Verification items for the finished model (mm, model axes). Face numbers are marked on the shaded views. A direction names the side the tool comes from. Give positions to 0.01 mm unless a question says otherwise; leave off trailing zeros. Write each loop counter-clockwise with the first axis right and the second up, starting at its lowest first coordinate (ties: lowest second). Pieces come first, ordered by that corner, then holes. Notation, with made-up numbers: (19, 77.5) - (38, 77.5) arc R28 cw to (38, 104.5) - close; hole circle Ø9 at (12, 24). An arc over 180 degrees is marked (long way). Answer as a JSON object with one key per item and string values. Group by question number.
Item 1: Draft check along Z on the marked faces 5, 6 and 7. Enter one of: +Z half, -Z half, draft (parallel to the pull), parting line (faces both ways), or undercut.
Item 2: Sectioned sample at C-C, the plane z = 15.5. Record the boundary of the cut face in (x, y), and give its area (3 significant figures).
Item 3: Sectioned sample at A-A, the plane x = 33. Record the boundary of the cut face in (y, z), and give its area (3 significant figures).
Item 4: Go/stop test with flat-tipped pins: pin 1 (5 mm diameter, centred on x = -39, y = 11, fed in from -Z); pin 2 (20 mm diameter, centred on y = 14.5, z = 8.5, fed in from +X); pin 3 (5 mm diameter, centred on y = 32, z = 1.5, fed in from -X). Record where each tip stops, or that it passes through.
Item 5: Sectioned sample at B-B, the plane y = 7.5. Record the boundary of the cut face in (x, z).
Item 6: Sectioned sample at D-D, the plane x = 19. Record the boundary of the cut face in (y, z).
Item 7: Tool access check on the marked faces 1, 2, 3 and 4. Record the directions out of +Z, -Z, +X, -X, +Y, -Y that give a thin tool (end or side, any length) a straight path to the whole face; none if there is none.
Item 8: Scan lines: line 1 along Z through (x, y) = (29, 29); line 2 along X through (y, z) = (28, -11.5); line 3 along X through (y, z) = (28, 23). Record each from-to range of solid material in increasing order. Write a range as [from, to].
```python
from build123d import *

# Parameters (mm, degrees)
SKETCH1_W               = 85
SKETCH1_H               = 60
BOSS_EXTRUDE1_DEPTH     = 40
SKETCH2_W               = 15
SKETCH2_H               = 40
CUT_EXTRUDE1_DEPTH      = 66.622023742
SKETCH3_W               = 20
SKETCH3_H               = 20
CUT_EXTRUDE2_DEPTH      = 10
CUT_EXTRUDE9_DEPTH      = 66.622023742
CUT_EXTRUDE9_DEPTH_BACK = 20
SKETCH6_W               = 20
SKETCH6_H               = 20
CUT_EXTRUDE10_DEPTH     = 10
CUT_EXTRUDE_THIN5_DEPTH = 56.733742024


with BuildPart() as part:
    # Sketch1 → Boss-Extrude1 (new body)
    with BuildSketch(Plane(origin=(0, 0, 0), x_dir=(1, 0, 0), z_dir=(0, 1, 0))):
        Rectangle(SKETCH1_W, SKETCH1_H)
    extrude(amount=BOSS_EXTRUDE1_DEPTH)

    # Sketch2 → Cut-Extrude1 (cut, through all)
    with BuildSketch(Plane(origin=(0, 40, 0), x_dir=(1, 0, 0), z_dir=(0, 1, 0))):
        with Locations((35, 0)):
            Rectangle(SKETCH2_W, SKETCH2_H)
    extrude(amount=-CUT_EXTRUDE1_DEPTH, mode=Mode.SUBTRACT)

    # Sketch3 → Cut-Extrude2 (cut)
    with BuildSketch(Plane(origin=(0, 40, 0), x_dir=(1, 0, 0), z_dir=(0, 1, 0))):
        with Locations((17.5, 0)):
            Rectangle(SKETCH3_W, SKETCH3_H)
    extrude(amount=-CUT_EXTRUDE2_DEPTH, mode=Mode.SUBTRACT)

    # Sketch4 → Cut-Extrude9 (cut, two sides: drawn at the far end of the back side and taken through both)
    with BuildSketch(Plane(origin=(0, 40, 0), x_dir=(1, 0, 0), z_dir=(0, 1, 0)).offset(-CUT_EXTRUDE9_DEPTH_BACK)):
        Polygon((7.5, 208.497084776), (7.5, 33.386024926), (7.5, -35.691822331), (7.5, -210.802882181), (-342.7221197, -210.802882181), (-342.7221197, 208.497084776), align=None)
    extrude(amount=CUT_EXTRUDE9_DEPTH + CUT_EXTRUDE9_DEPTH_BACK, mode=Mode.SUBTRACT)

    # Sketch6 → Cut-Extrude10 (cut)
    with BuildSketch(Plane.ZY.offset(42.5)):
        with Locations((0, 10)):
            Rectangle(SKETCH6_W, SKETCH6_H)
    extrude(amount=-CUT_EXTRUDE10_DEPTH, mode=Mode.SUBTRACT)

    # Sketch9 → Cut-Extrude-Thin5 (cut, through all)
    with BuildSketch(Plane(origin=(0, 20, 0), x_dir=(1, 0, 0), z_dir=(0, 1, 0))):
        Polygon((-17.5, 30.102443268), (-42.5, 20), (-46.246635858, 29.271608261), (-21.246635858, 39.374051529), align=None)
        Polygon((-42.5, -20), (-17.5, -30), (-21.213906764, -39.284766909), (-46.213906764, -29.284766909), align=None)
    extrude(amount=-CUT_EXTRUDE_THIN5_DEPTH, mode=Mode.SUBTRACT)


solid = part.part
```
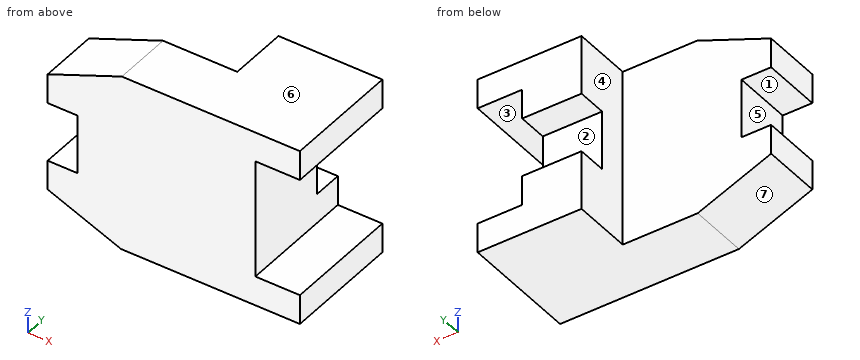
Geometry check:
{
 "1": {"face 5": "undercut", "face 6": "+Z half", "face 7": "-Z half"},
 "2": {"outline": "(-42.5, 0) - (27.5, 0) - (27.5, 40) - (7.5, 40) - (7.5, 20) - (-42.5, 20) - close", "area": "1,800 mm^2"},
 "3": {"outline": "(0, -30) - (40, -30) - (40, -20) - (0, -20) - close; (0, 20) - (40, 20) - (40, 30) - (0, 30) - close", "area": "800 mm^2"},
 "4": {"pin 1": "z = -22.42", "pin 2": "x = 27.5", "pin 3": "x = 7.5"},
 "5": {"outline": "(-42.5, -20) - (-17.75, -30) - (42.5, -30) - (42.5, -20) - (27.5, -20) - (27.5, 20) - (42.5, 20) - (42.5, 30) - (-17.5, 30) - (-42.5, 20) - (-42.5, 10) - (-32.5, 10) - (-32.5, -10) - (-42.5, -10) - close"},
 "6": {"outline": "(0, -30) - (40, -30) - (40, -10) - (30, -10) - (30, 10) - (40, 10) - (40, 30) - (0, 30) - close"},
 "7": {"face 1": "-X, +Y, -Y", "face 2": "+X, -X, +Y", "face 3": "+X, +Y, -Y", "face 4": "+Z, -Z, -X, +Y"},
 "8": {"line 1": "[-30, -20], [20, 30]", "line 2": "[7.5, 27.5]", "line 3": "[7.5, 42.5]"}
}
